Study the drawing (mm; zero at the part's minimum x, y, z) and answer. Give positions to 0.01 mm unless a question says otherwise; leave off trailing zeros. Loops run counter-clockwise (first coordinate to the right, second up) from the corner with the lowest first, then second, coordinate; pieces in that order, holes last. Notation, with made-up numbers: (-0.5, 66.25) - (19.5, 66.25) arc R8 ccw to (19.5, 75.25) - close; hole circle Ø2 at (14.25, 28). An arc over 180 degrees is marked (long way). Write item = value, one per line. Start each with the question number.
1) The part is cut by section C-C on z = 2.1. Write down the section's boundary in (x, y).
2) The part is cut by section A-A on y = 25. Write down the section's boundary in (x, z), plus the area to 3 significant figures.
3) The part is cut by section D-D on x = 50. Write down the section's boundary in (y, z).
4) Consider probe 1 along Y at (x, z) = (10, 2.75); probe 2 along X at (y, z) = (22.75, 3.15); probe 3 along X at (y, z) = (13.5, 3.6). Determine where each line is inside the solid, lowest interval first.
5) The part is cut by section B-B on x = 10. Write down the section's boundary in (y, z), plus the area to 3 significant figures.
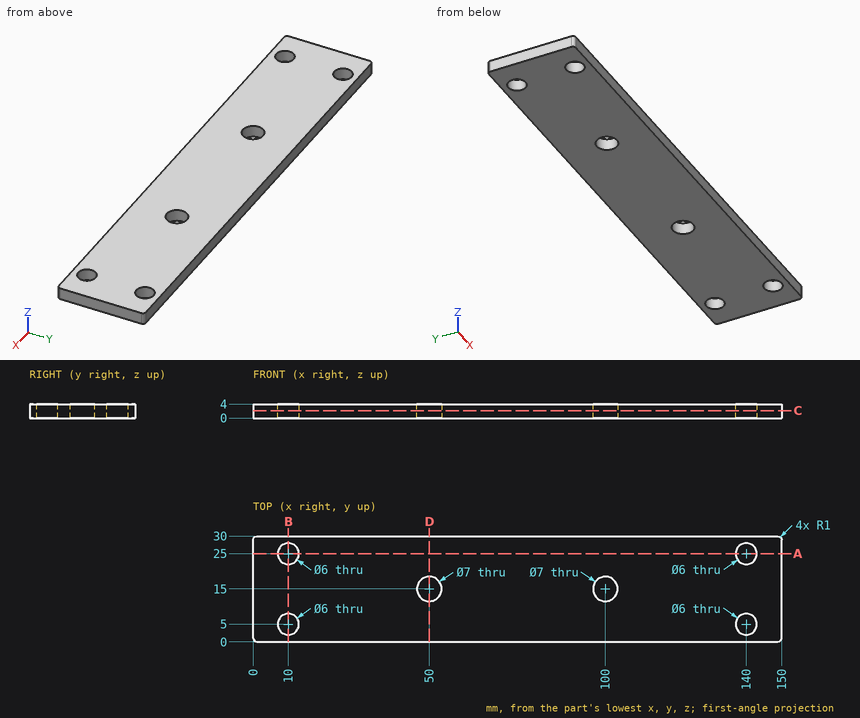
Answer below:
q1.outline = (0, 1) arc R1 ccw to (1, 0) - (149, 0) arc R1 ccw to (150, 1) - (150, 29) arc R1 ccw to (149, 30) - (1, 30) arc R1 ccw to (0, 29) - close; hole circle Ø6 at (10, 5); hole circle Ø6 at (10, 25); hole circle Ø7 at (50, 15); hole circle Ø7 at (100, 15); hole circle Ø6 at (140, 5); hole circle Ø6 at (140, 25)
q2.outline = (0, 0) - (7, 0) - (7, 4) - (0, 4) - close; (13, 0) - (137, 0) - (137, 4) - (13, 4) - close; (143, 0) - (150, 0) - (150, 4) - (143, 4) - close
q2.area = 552 mm2
q3.outline = (0, 0) - (11.5, 0) - (11.5, 4) - (0, 4) - close; (18.5, 0) - (30, 0) - (30, 4) - (18.5, 4) - close
q4.probe_1 = 0 to 2, 8 to 22, 28 to 30
q4.probe_2 = 0 to 8.02, 11.98 to 138.02, 141.98 to 150
q4.probe_3 = 0 to 46.84, 53.16 to 96.84, 103.16 to 150
q5.outline = (0, 0) - (2, 0) - (2, 4) - (0, 4) - close; (8, 0) - (22, 0) - (22, 4) - (8, 4) - close; (28, 0) - (30, 0) - (30, 4) - (28, 4) - close
q5.area = 72.0 mm2
